Can you work these out from the drawing? Everything is in mm from the part's minimum corner. A direction names the side the tool comes from. Coordinates: 2 decimals unless noted, no trailing zeros. Order: outer loops, then holes, each group sorted by start corner. A loop starts at its lowest first (then second) coordinate and runs counter-clockwise, first axis right, second up. Notation, with made-up numbers: (13.25, 78.5) - (26.25, 78.5) arc R11 ccw to (26.25, 86.5) - close; hole circle Ø7 at (52.25, -35.5). An arc over 180 degrees is marked (long way). Use one line per item in the form item = value. Start each with the question number.
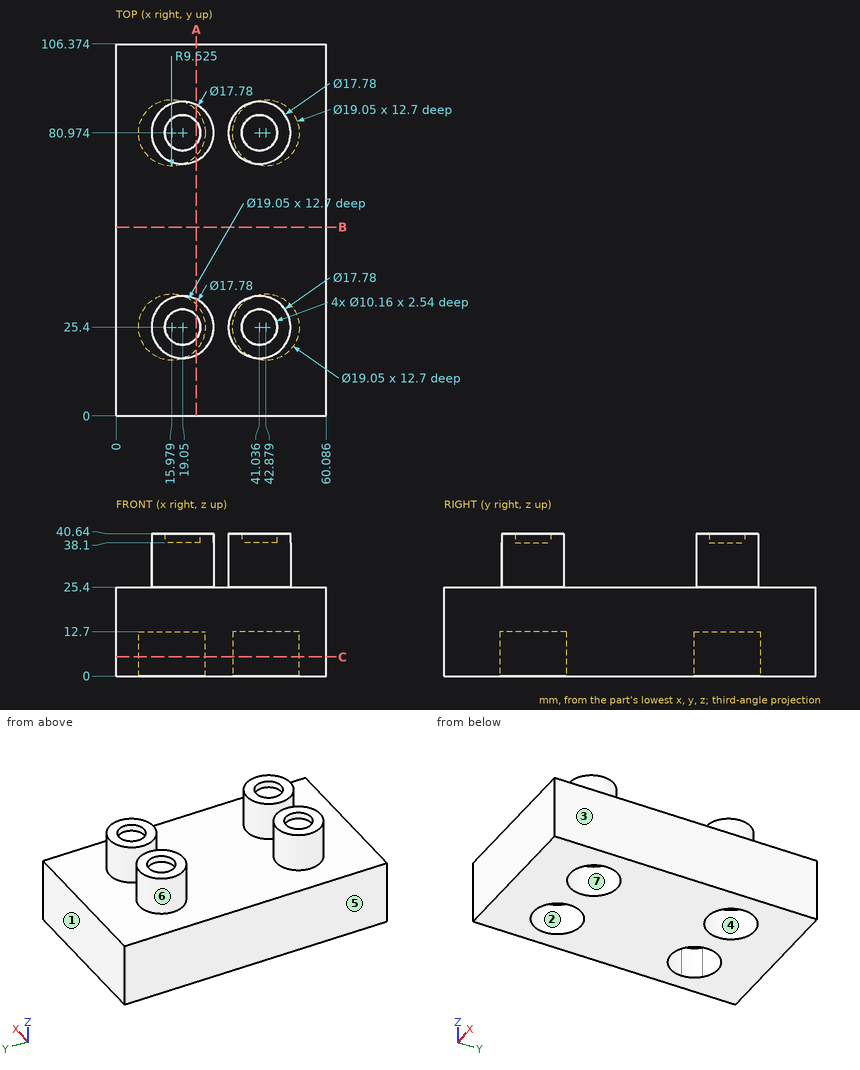
1) Which directions (+Z, -Z, +X, -X, +Y, -Y) give clear straight access to the entire face, cutting with the end or side of a thin tool? Please do the marked faces 5, 6 and 7.
2) Suppose I cut it at B-B, the plane y = 54. List the corners of the cut face in (x, z) for me, then the cut area to 3 significant figures.
3) Suppose I cut it at A-A, the plane x = 23. List the corners of the cut face in (y, z) for me (1 decimal), then the cut area to 3 significant figures.
4) For pin 1 (9.5 mm diameter, centred on x = 44.5, y = 80.5, fed in from -Z); pin 2 (8 mm diameter, centred on x = 41.04, y = 80.97, fed in from +Z); pin 3 (10 mm diameter, centred on x = 51, y = 12.5, fed in from +Z), each with a flat end and sliding along its axis, tell me the tip position at first contact or that it passes through.
5) Suppose I cut it at C-C, the plane z = 5.5. Give the number of separate pieces and of enclosed holes in the cut face, then the cut area to 3 significant figures.
6) If we mould it in two halves opening along X, with no side actions, what happens to the marked faces 1, 2, 3 and 4? For each: pulls with the +X half, pulls with the -X half, needs draft (parallel to the pull), parting line crosses it, or undercut.
7) I need wall thicknesses on probe 1 along X at (y, z) = (25, 7) (1 decimal); probe 2 along X at (y, z) = (25.4, 39); probe 3 along X at (y, z) = (25, 39) (1 decimal). Which ranges of each line are inside material? Lowest first, please. Write a range as [from, to].
From the geometry:
q1.face_5 = +Z, -Z, -X, +Y, -Y
q1.face_6 = +Z
q1.face_7 = -Z
q2.outline = (0, 0) - (60.09, 0) - (60.09, 25.4) - (0, 25.4) - close
q2.area = 1,530 mm2
q3.outline = (0, 0) - (19, 0) - (19, 12.7) - (31.8, 12.7) - (31.8, 0) - (74.5, 0) - (74.5, 12.7) - (87.4, 12.7) - (87.4, 0) - (106.4, 0) - (106.4, 25.4) - (88.9, 25.4) - (88.9, 40.6) - (84.2, 40.6) - (84.2, 38.1) - (77.8, 38.1) - (77.8, 40.6) - (73, 40.6) - (73, 25.4) - (33.4, 25.4) - (33.4, 40.6) - (28.6, 40.6) - (28.6, 38.1) - (22.2, 38.1) - (22.2, 40.6) - (17.4, 40.6) - (17.4, 25.4) - (0, 25.4) - close
q3.area = 2,830 mm2
q4.pin_1 = 12.7
q4.pin_2 = 38.1
q4.pin_3 = 25.4
q5.separate_pieces = 1
q5.enclosed_holes = 4
q5.area = 5,250 mm2
q6.face_1 = needs draft
q6.face_2 = undercut
q6.face_3 = pulls with the +X half
q6.face_4 = undercut
q7.probe_1 = [0, 6.5], [25.5, 33.4], [52.4, 60.1]
q7.probe_2 = [10.16, 13.97], [24.13, 27.94], [32.15, 35.96], [46.12, 49.93]
q7.probe_3 = [10.2, 14], [24.1, 27.9], [32.2, 36], [46.1, 49.9]
